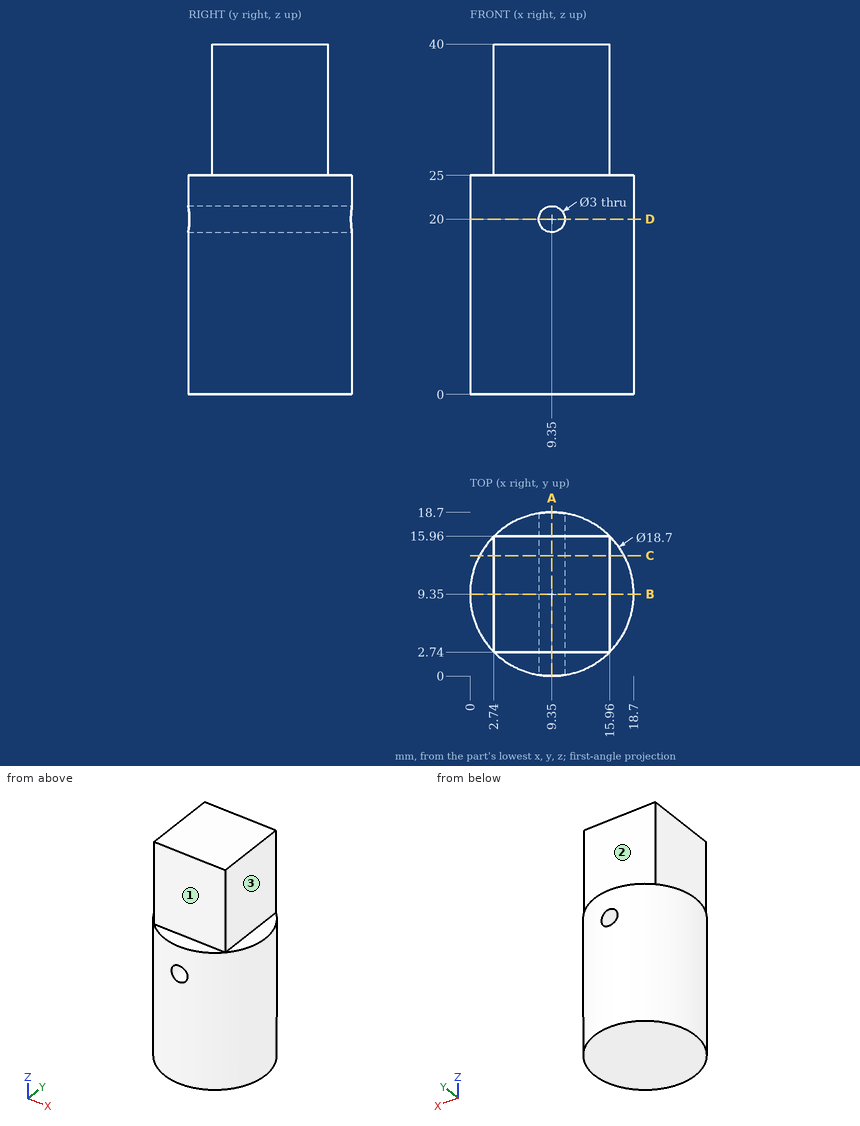
Can you work these out from the drawing? Everything is in mm from the part's minimum corner. A direction names the side the tool comes from. Coordinates: 2 decimals unless noted, no trailing zeros. Order: outer loops, then holes, each group sorted by start corner. A loop starts at its lowest first (then second) coordinate and runs counter-clockwise, first axis right, second up. Notation, with made-up numbers: (74.25, 33.5) -> (85.25, 33.5) arc R32 cw to (85.25, 70.5) -> close; hole circle Ø11 at (43.25, 11.25). An arc over 180 degrees is marked (long way). Use one line per item in the form item = value.
Q1. Imagine slicing it at B-B, the plane y = 9.35. List the corners of the cut face in (x, z) for me.
From the geometry:
outline = (0, 0) -> (18.7, 0) -> (18.7, 25) -> (15.96, 25) -> (15.96, 40) -> (2.74, 40) -> (2.74, 25) -> (0, 25) -> close; hole circle Ø3 at (9.35, 20)
Q2. I need wall thicknesses on L1, parallel to Z at x = 9.35, y = 9; L2, parallel to Y at x = 4.75, z = 25.5. Which ranges of each line are inside material? Lowest first, please.
From the geometry:
L1 = 0 to 18.5, 21.5 to 40
L2 = 2.74 to 15.96
Q3. Which directions (+Z, -Z, +X, -X, +Y, -Y) give clear straight access to the entire face, cutting with the end or side of a thin tool? Please do the marked faces 1, 2 and 3.
From the geometry:
face_1 = +Z, +X, -X, -Y
face_2 = +Z, +X, -X, +Y
face_3 = +Z, +X, +Y, -Y
Q4. Will these pins go through, and if not, where does the flat tip stop? P1, Ø3, axis at y = 12.5, z = 32.5, coming from the -X side; P2, Ø10, axis at y = 4, z = 17, coming from the +X side; P3, Ø4, axis at x = 10, z = 35.5, coming from the +Y side.
From the geometry:
P1 = 2.74
P2 = 18.69
P3 = 15.96
Q5. Imagine slicing it at D-D, the plane z = 20. List the corners of the cut face in (x, y) for me.
From the geometry:
outline = (7.85, 0.12) -> (7.85, 18.58) arc R9.35 ccw to start; (10.85, 0.12) arc R9.35 ccw to (10.85, 18.58) -> close
Q6. Imagine slicing it at A-A, the plane x = 9.35. List the corners of the cut face in (y, z) for me.
From the geometry:
outline = (0, 0) -> (18.7, 0) -> (18.7, 18.5) -> (0, 18.5) -> close; (0, 21.5) -> (18.7, 21.5) -> (18.7, 25) -> (15.96, 25) -> (15.96, 40) -> (2.74, 40) -> (2.74, 25) -> (0, 25) -> close
Q7. Imagine slicing it at C-C, the plane y = 13.75. List the corners of the cut face in (x, z) for me.
From the geometry:
outline = (1.1, 0) -> (17.6, 0) -> (17.6, 25) -> (15.96, 25) -> (15.96, 40) -> (2.74, 40) -> (2.74, 25) -> (1.1, 25) -> close; hole circle Ø3 at (9.35, 20)
